```python
from build123d import *

# Parameters (mm, degrees)
F0_W     = 260.35
F0_H     = 196.85
F0_W_2   = 228.6
F0_H_2   = 101.6
F0_R     = 31.75
F1_DEPTH = 9.525


with BuildPart() as f1:
    # F0 (on Top) → F1 (new body)
    with BuildSketch(Plane.XY):
        with Locations((130.175, -98.425)):
            Rectangle(F0_W, F0_H)
        with Locations((130.175, -136.9441)):
            Rectangle(F0_W_2, F0_H_2, mode=Mode.SUBTRACT)
        with Locations((47.625, -45.2882)):
            Circle(F0_R, mode=Mode.SUBTRACT)
        with Locations((130.175, -45.2882)):
            Circle(F0_R, mode=Mode.SUBTRACT)
        with Locations((212.725, -45.2882)):
            Circle(F0_R, mode=Mode.SUBTRACT)
    extrude(amount=F1_DEPTH)


solid = f1.part
```
Design review of the part built by this model. Coordinates are the model's own, in mm. A direction names the side the tool comes from. Round coordinates to 2 decimals unless told otherwise and drop trailing zeros. Write each loop counter-clockwise with the first axis right and the second up, starting at its lowest first coordinate (ties: lowest second). Pieces come first, ordered by that corner, then holes.
Item 1: For probe 1 along X at (y, z) = (-45, 5); probe 2 along X at (y, z) = (-139.5, 1.25) (3 decimals); probe 3 along Y at (x, z) = (112.5, 2.5), list the stretches that pass through material, from the lowest coordinate up.
Item 2: For faces 1 (the flat face through (260.35, -100, 5)), 2 (the flat face through (129, -187.744, 5)), list the 3-axis set-ups (+Z, -Z, +X, -X, +Y, -Y) from which the entire face can be reached by the end or side of a thin tool; tool diameter is ignored.
Item 3: We need section A-A on x = 89.5. Write out the cut boundary in (y, z) (3 decimals), and give its area (3 significant figures).
Item 4: Clearance check with a flat-ended pin moving along its axis: pin 1 Ø2 at (x, z) = (44.5, 3) entering from +Y. State where the tip first meets the part, or that it passes through.
Item 5: We need section C-C on y = -55. Write out the cut boundary in (x, z) (3 decimals), and give its area (3 significant figures).
Item 6: We need section B-B on y = -116. Write out the cut boundary in (x, z) (3 decimals).
Item 7: We need section D-D on x = 152.5. Write out the cut boundary in (y, z) (3 decimals), and give its area (3 significant figures).
Item 8: The part is to be moulded in two halves that separate along Y. For faces 3 (the flat face through (15.875, -138, 5)), 4 (the flat face through (244.475, -138, 5)), 5 (the flat face through (128, 0, 5)), 6 (the flat face through (139, -76, 0)), say which applies: +Y half, -Y half, draft (parallel to the pull), parting line (faces both ways), or undercut.
Returned:
1. probe 1: x = 0 to 15.88, 79.37 to 98.43, 161.92 to 180.98, 244.47 to 260.35
1. probe 2: x = 0 to 15.875, 244.475 to 260.35
1. probe 3: y = -196.85 to -187.74, -86.14 to -71.66, -18.91 to 0
2. face 1: +Z, -Z, +X, +Y, -Y
2. face 2: +Z, -Z
3. outline: (-196.85, 0) - (-187.744, 0) - (-187.744, 9.525) - (-196.85, 9.525) - close; (-86.144, 0) - (0, 0) - (0, 9.525) - (-86.144, 9.525) - close
3. area: 907 mm2
4. pin 1: stops at y = 0
5. outline: (0, 0) - (17.397, 0) - (17.397, 9.525) - (0, 9.525) - close; (77.853, 0) - (99.947, 0) - (99.947, 9.525) - (77.853, 9.525) - close; (160.403, 0) - (182.497, 0) - (182.497, 9.525) - (160.403, 9.525) - close; (242.953, 0) - (260.35, 0) - (260.35, 9.525) - (242.953, 9.525) - close
5. area: 752 mm2
6. outline: (0, 0) - (15.875, 0) - (15.875, 9.525) - (0, 9.525) - close; (244.475, 0) - (260.35, 0) - (260.35, 9.525) - (244.475, 9.525) - close
7. outline: (-196.85, 0) - (-187.744, 0) - (-187.744, 9.525) - (-196.85, 9.525) - close; (-86.144, 0) - (-67.864, 0) - (-67.864, 9.525) - (-86.144, 9.525) - close; (-22.713, 0) - (0, 0) - (0, 9.525) - (-22.713, 9.525) - close
7. area: 477 mm2
8. face 3: undercut
8. face 4: undercut
8. face 5: +Y half
8. face 6: draft
